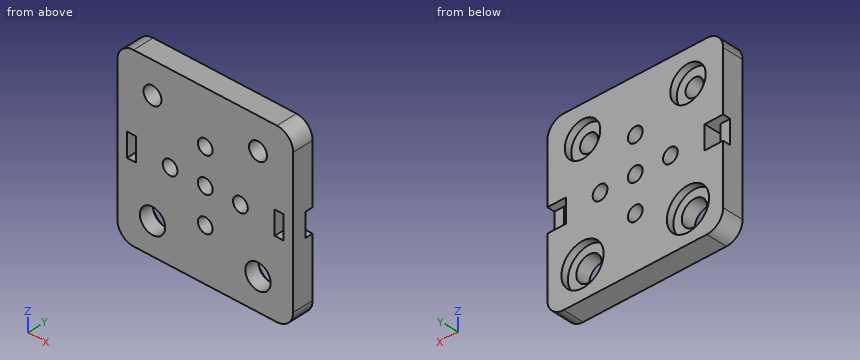
```python
from build123d import *

# Parameters (mm, degrees)
SKETCH1_R             = 3.6
SKETCH1_R_2           = 2.55
BOSS_EXTRUDE1_DEPTH   = 6
M5X0_8_TAPPED_HOLE1_D = 4.2
SKETCH2_R             = 6
SKETCH2_R_2           = 5.05
CUT_EXTRUDE1_DEPTH    = 2
SKETCH5_W             = 5.25
SKETCH5_H             = 6.7
CUT_EXTRUDE2_DEPTH    = 2.18
SKETCH6_W             = 2.5
SKETCH6_H             = 6.7
CUT_EXTRUDE3_DEPTH    = 4.82


with BuildPart() as part:
    # Sketch1 → Boss-Extrude1 (new body)
    with BuildSketch(Plane(origin=(0, 0, 0), x_dir=(1, 0, 0), z_dir=(0, 1, 0))):
        with BuildLine():
            Line((20.365, -25), (-20.365, -25))
            ThreePointArc((-20.365, -25), (-23.642439931, -23.642439931), (-25, -20.365))
            Line((-25, -20.365), (-25, 20.365))
            ThreePointArc((-25, 20.365), (-23.642439931, 23.642439931), (-20.365, 25))
            Line((-20.365, 25), (20.365, 25))
            ThreePointArc((20.365, 25), (23.642439931, 23.642439931), (25, 20.365))
            Line((25, 20.365), (25, -20.365))
            ThreePointArc((25, -20.365), (23.642439931, -23.642439931), (20.365, -25))
        make_face()
        with Locations((-15, 15.95)):
            Circle(SKETCH1_R, mode=Mode.SUBTRACT)
        with Locations((15, 15.95)):
            Circle(SKETCH1_R, mode=Mode.SUBTRACT)
        with Locations((15, -15.95)):
            Circle(SKETCH1_R_2, mode=Mode.SUBTRACT)
        with Locations((-15, -15.95)):
            Circle(SKETCH1_R_2, mode=Mode.SUBTRACT)
    extrude(amount=BOSS_EXTRUDE1_DEPTH)

    # M5x0.8 Tapped Hole1 (through all)
    with Locations(Plane(origin=(0, 6, 0), x_dir=(1, 0, 0), z_dir=(0, 1, 0))):
        with Locations((0, 10), (-10, 0), (0, 0), (0, -10), (10, 0)):
            Hole(M5X0_8_TAPPED_HOLE1_D / 2)

    # Sketch2 → Cut-Extrude1 (cut)
    with BuildSketch(Plane(origin=(0, 6, 0), x_dir=(1, 0, 0), z_dir=(0, 1, 0))):
        with Locations((-15, 15.95)):
            Circle(SKETCH2_R)
        with Locations((15, 15.95)):
            Circle(SKETCH2_R)
        with Locations((15, -15.95)):
            Circle(SKETCH2_R_2)
        with Locations((-15, -15.95)):
            Circle(SKETCH2_R_2)
    extrude(amount=-CUT_EXTRUDE1_DEPTH, mode=Mode.SUBTRACT)

    # Sketch5 → Cut-Extrude2 (cut)
    with BuildSketch(Plane(origin=(0, 6, 0), x_dir=(1, 0, 0), z_dir=(0, 1, 0))):
        with Locations((-22.375, 0)):
            Rectangle(SKETCH5_W, SKETCH5_H)
        with Locations((22.375, 0)):
            Rectangle(SKETCH5_W, SKETCH5_H)
    extrude(amount=-CUT_EXTRUDE2_DEPTH, mode=Mode.SUBTRACT)

    # Sketch6 → Cut-Extrude3 (cut, through all)
    with BuildSketch(Plane(origin=(0, 3.82, 0), x_dir=(1, 0, 0), z_dir=(0, 1, 0))):
        with Locations((-21, 0)):
            Rectangle(SKETCH6_W, SKETCH6_H)
        with Locations((21, 0)):
            Rectangle(SKETCH6_W, SKETCH6_H)
    extrude(amount=-CUT_EXTRUDE3_DEPTH, mode=Mode.SUBTRACT)


solid = part.part
```
Check sheet for the modelled part. Datum: model origin and axes. Units: mm. Round coordinates to 2 decimals unless told otherwise and drop trailing zeros. Order: outer loops, then holes, each group sorted by start corner. A loop starts at its lowest first (then second) coordinate and runs counter-clockwise, first axis right, second up.
1) Section check B-B (z = 10). Record the boundary of the cut face in (x, y).
2) Section check C-C (y = 2.15). Give the number of separate pieces and of enclosed holes in the cut face, and give its area (3 significant figures).
3) Scan lines: line 1 (X direction, y = 3.7, z = -16); line 2 (X direction, y = 2.75, z = 16); line 3 (Z direction, x = 0, y = 3). Record each from-to range of solid material in increasing order.
4) Section check D-D (z = 15.95). Record the boundary of the cut face in (x, y), and give its area (3 significant figures).
5) Go/stop test with flat-tipped pins: pin 1 Ø2 at (x, z) = (-23, 1.5) entering from +Y; pin 2 Ø3.5 at (x, z) = (0, 10) entering from -Y; pin 3 Ø6 at (x, z) = (-12.5, -17.5) entering from +Y. Record where each tip stops, or that it passes through.
6) Section check A-A (x = 0). Record the boundary of the cut face in (y, z).
Result:
1. outline: (-25, 0) - (-2.1, 0) - (-2.1, 6) - (-25, 6) - close; (2.1, 0) - (25, 0) - (25, 6) - (2.1, 6) - close
2. separate pieces: 1
2. enclosed holes: 11
2. area: 2,260 mm2
3. line 1: x = -25 to -18.6, -11.4 to 11.4, 18.6 to 25
3. line 2: x = -25 to -17.55, -12.45 to 12.45, 17.55 to 25
3. line 3: z = -25 to -12.1, -7.9 to -2.1, 2.1 to 7.9, 12.1 to 25
4. outline: (-25, 0) - (-17.55, 0) - (-17.55, 4) - (-20.05, 4) - (-20.05, 6) - (-25, 6) - close; (-12.45, 0) - (12.45, 0) - (12.45, 4) - (9.95, 4) - (9.95, 6) - (-9.95, 6) - (-9.95, 4) - (-12.45, 4) - close; (17.55, 0) - (25, 0) - (25, 6) - (20.05, 6) - (20.05, 4) - (17.55, 4) - close
4. area: 219 mm2
5. pin 1: stops at y = 3.82
5. pin 2: passes through
5. pin 3: stops at y = 4
6. outline: (0, -25) - (6, -25) - (6, -12.1) - (0, -12.1) - close; (0, -7.9) - (6, -7.9) - (6, -2.1) - (0, -2.1) - close; (0, 2.1) - (6, 2.1) - (6, 7.9) - (0, 7.9) - close; (0, 12.1) - (6, 12.1) - (6, 25) - (0, 25) - close
